from build123d import *

# Parameters (mm, degrees)
F0_W           = 400
F0_H           = 400
F1_DEPTH       = 95
F3_D           = 17.5
F3_CBORE_D     = 26
F3_CBORE_DEPTH = 17
F5_D           = 21.5
F5_CBORE_D     = 32
F5_CBORE_DEPTH = 21


with BuildPart() as f1:
    # F0 (on Top) → F1 (new body)
    with BuildSketch(Plane.XY):
        Rectangle(F0_W, F0_H)
    extrude(amount=F1_DEPTH)

    # F3 (through all)
    with Locations(Plane(origin=(0, 0, 0), x_dir=(1, 0, 0), z_dir=(0, 0, -1))):
        with Locations((0, 0), (0, 50), (-50, 0), (0, -50), (50, 0)):
            CounterBoreHole(F3_D / 2, F3_CBORE_D / 2, F3_CBORE_DEPTH)

    # F5 (through all)
    with Locations(Plane.XY.offset(95)):
        with Locations((-125, 125), (125, 125), (-125, -125), (125, -125)):
            CounterBoreHole(F5_D / 2, F5_CBORE_D / 2, F5_CBORE_DEPTH)


solid = f1.part
Design review of the part built by this model. Coordinates are the model's own, in mm. A direction names the side the tool comes from. Round coordinates to 2 decimals unless told otherwise and drop trailing zeros. Order: outer loops, then holes, each group sorted by start corner. A loop starts at its lowest first (then second) coordinate and runs counter-clockwise, first axis right, second up. Notation, with made-up numbers: M -10.5,4 L 2.5,4 A21 cw 2.5,12 Z; hole C 53,-9.5 d6. An arc over 180 degrees is marked long. Answer as CSV lines item,"result". Start each with the question number.
1) Add section D-D (y = -125). Give the boundary of the cut face in (x, z), then the cut area to 3 significant figures.
2) For pin 1 Ø4 at (x, y) = (115.5, 123) entering from +Z; pin 2 Ø23.5 at (x, y) = (0, 0) entering from -Z; pin 3 Ø16 at (x, y) = (0, -50) entering from +Z, all flat-tipped, find the tip position at first contact; note any pin that passes through.
3) The part is to be moulded in two halves that separate along X. For faces 1 (the face through (-3, 200, 47)), 2 (the face through (-200, -3, 47)), 3 (the face through (8.5, 52.7, 17)), 4 (the face through (200, -3, 47)), say which applies: +X half, -X half, draft (parallel to the pull), parting line (faces both ways), or undercut.
4) Tool access review of faces 5 (the face through (56.944, 5.324, 56.546)), 6 (the face through (-62.987, -0.572, 8.381)), 7 (the face through (135.4, 121.7, 74)): name each direction out of +Z, -Z, +X, -X, +Y, -Y from which nothing blocks a thin tool from reaching the whole face with its end or side.
5) Wall thickness on line 1 along Y through (x, z) = (-125, 16.5); line 2 along Y through (x, z) = (0, 75.5); line 3 along X through (y, z) = (8, 55): over which ranges is each line inside the solid? List them lowest first. Write a range as [from, to].
6) Add section A-A (y = 50). Give the boundary of the cut face in (x, z), then the cut area to 3 significant figures.
7) Add section C-C (z = 26). Give the number of separate pieces and of enclosed holes in the cut face, then the cut area to 3 significant figures.
Resolved:
1,outline,"M -200,0 L -135.75,0 L -135.75,74 L -141,74 L -141,95 L -200,95 Z; M -114.25,0 L 114.25,0 L 114.25,74 L 109,74 L 109,95 L -109,95 L -109,74 L -114.25,74 Z; M 135.75,0 L 200,0 L 200,95 L 141,95 L 141,74 L 135.75,74 Z"
1,area,"33,500 mm^2"
2,pin 1,"z = 74"
2,pin 2,"z = 17"
2,pin 3,"through"
3,face 1,"draft"
3,face 2,"-X half"
3,face 3,"undercut"
3,face 4,"+X half"
4,face 5,"+Z, -Z"
4,face 6,"-Z"
4,face 7,"+Z"
5,line 1,"[-200, -135.75], [-114.25, 114.25], [135.75, 200]"
5,line 2,"[-200, -58.75], [-41.25, -8.75], [8.75, 41.25], [58.75, 200]"
5,line 3,"[-200, -53.54], [-46.46, -3.54], [3.54, 46.46], [53.54, 200]"
6,outline,"M -200,0 L -13,0 L -13,17 L -8.75,17 L -8.75,95 L -200,95 Z; M 8.75,17 L 13,17 L 13,0 L 200,0 L 200,95 L 8.75,95 Z"
6,area,"36,200 mm^2"
7,separate pieces,"1"
7,enclosed holes,"9"
7,area,"157,000 mm^2"
